Geometry: final body of the model. Coordinates: model frame, mm. Face numbers are marked on the shaded views. Give positions to 0.01 mm unless a question says otherwise; leave off trailing zeros. Order: outer loops, then holes, each group sorted by start corner. A loop starts at its lowest first (then second) coordinate and runs counter-clockwise, first axis right, second up. Notation, with made-up numbers: (3, 12.5) - (9, 12.5) arc R11 cw to (9, 19.5) - close; hole circle Ø1 at (85.25, 4). An arc over 180 degrees is marked (long way). Use one line per item in the form item = value.
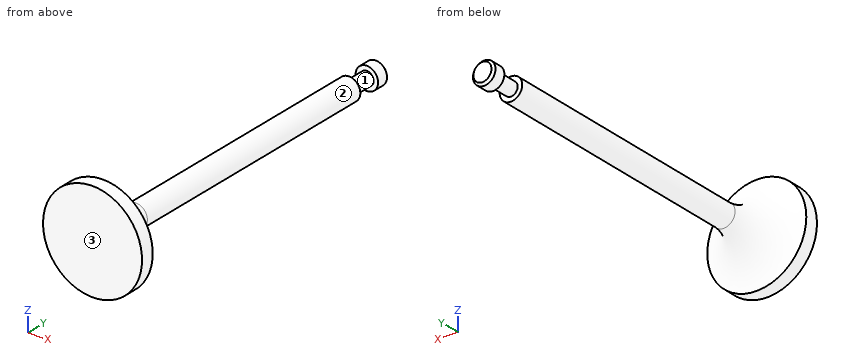
from build123d import *

# Parameters (mm, degrees)
CHAMFER1_SIZE = 0.5


with BuildPart() as part:
    # Sketch1 → Revolve1 (revolve)
    with BuildSketch(Plane.XY, mode=Mode.PRIVATE) as revolve1_sk:
        with BuildLine():
            Line((0, 0), (11, 0))
            Line((11, 0), (11, 3))
            ThreePointArc((11, 3), (5.117826553, 6.121629363), (2.5, 12.244661169))
            Line((2.5, 12.244661169), (2.5, 72))
            Line((2.5, 72), (1.5, 72))
            Line((1.5, 72), (1.5, 77))
            Line((1.5, 77), (2.5, 77))
            Line((2.5, 77), (2.5, 80))
            Line((2.5, 80), (0, 80))
            Line((0, 80), (0, 0))
        make_face()
    revolve(revolve1_sk.sketch.rotate(Axis((0, 80, 0), (0, -1, 0)), 180), axis=Axis((0, 80, 0), (0, -1, 0)))

    # Chamfer1
    chamfer1_edges = [part.edges().sort_by_distance(p)[0] for p in [
        (2.5, 80, 0),
    ]]
    chamfer(chamfer1_edges, length=CHAMFER1_SIZE)


solid = part.part
(1) Cut plane B-B on z = 0. Output: boundary loops of the cut face in (x, y), plus the area to 3 significant figures.
Computed values:
outline = (-11, 0) - (11, 0) - (11, 3) arc R10 cw to (2.5, 12.24) - (2.5, 72) - (1.5, 72) - (1.5, 77) - (2.5, 77) - (2.5, 79.5) - (2, 80) - (-2, 80) - (-2.5, 79.5) - (-2.5, 77) - (-1.5, 77) - (-1.5, 72) - (-2.5, 72) - (-2.5, 12.24) arc R10 cw to (-11, 3) - close
area = 481 mm²
(2) Contact query for flat-ended pins moving along their axis: pin 1 Ø10 at (y, z) = (36.5, -0.5) entering from -X; pin 2 Ø2.5 at (x, z) = (1, -0.5) entering from -Y; pin 3 Ø3 at (x, y) = (2.5, 33) entering from +Z; pin 4 Ø10 at (x, z) = (-5.5, 5) entering from +Y. Output: stop coordinate, or through.
Computed values:
pin_1 = -2.5
pin_2 = 0
pin_3 = 2.29
pin_4 = 79.57
(3) Cut plane A-A on x = 0. Output: boundary loops of the cut face in (y, z), plus the area to 3 significant figures.
Computed values:
outline = (0, -11) - (3, -11) arc R10 cw to (12.24, -2.5) - (72, -2.5) - (72, -1.5) - (77, -1.5) - (77, -2.5) - (79.5, -2.5) - (80, -2) - (80, 2) - (79.5, 2.5) - (77, 2.5) - (77, 1.5) - (72, 1.5) - (72, 2.5) - (12.24, 2.5) arc R10 cw to (3, 11) - (0, 11) - close
area = 481 mm²
(4) Pull-direction query (Y, two-part tool) for the marked faces 1, 2 and 3; classes: released by +Y, released by -Y, zero draft, split by the parting line, or undercut.
Computed values:
face_1 = undercut
face_2 = zero draft
face_3 = released by -Y
(5) Ray query, line 1 along Y through (x, z) = (1.25, 1.5); line 2 along X through (y, z) = (11.5, -1.5); line 3 along Y through (x, z) = (-4, -3.5). Return the intervals inside material, ascending.
Computed values:
line_1 = 0 to 72, 77 to 80
line_2 = -2.09 to 2.09
line_3 = 0 to 5.91
(6) Cut plane C-C on y = 55. Output: boundary loops of the cut face in (x, z), plus the area to 3 significant figures.
Computed values:
outline = circle Ø5 at (0, 0)
area = 19.6 mm²
